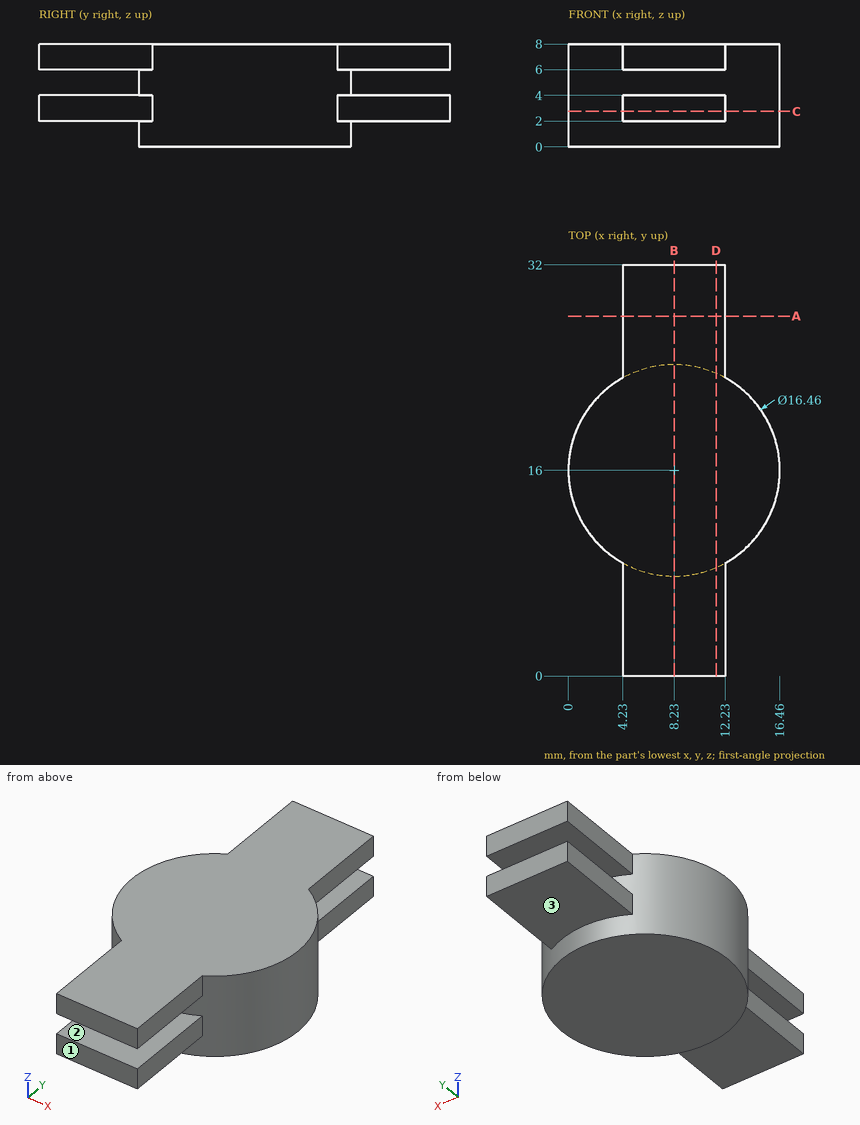
Geometry: see drawing. Coordinates: mm, zero at the bounding-box minimum. Give positions to 0.01 mm unless a question says otherwise; leave off trailing zeros. Write each loop counter-clockwise with the first axis right and the second up, starting at its lowest first coordinate (ties: lowest second). Pieces come first, ordered by that corner, then holes. Notation, with made-up numbers: M 51,74 L 65,74 A35 ccw 65,111 Z; hole C 87.25,0.25 d6. An arc over 180 degrees is marked long. Answer in a Markdown table with one row per item. Add a question column.
(1) Mould query, pull axis Z, two halves, no side actions, for the marked faces 1, 2 and 3. Classes: +Z half, -Z half, draft (parallel to the pull), parting line (faces both ways), or undercut.
(2) Section A-A on y = 28. Return loops of the section in (x, z).
(3) Section B-B on x = 8.23. Return loops of the section in (y, z), and give its area (3 significant figures).
(4) Section C-C on z = 2.75. Return loops of the section in (x, y).
(5) Section D-D on x = 11.5. Return loops of the section in (y, z).
(6) Ray query, line 1 (Z direction, x = 8, y = 25.5); line 2 (X direction, y = 29, z = 3); line 3 (Y direction, x = 8.25, z = 1.25). Return the intervals inside material, ascending.
(7) First-contact query: pin 1 (1.6 mm diameter, centred on y = 3.5, z = 7.5, fed in from +X); pin 2 (1 mm diameter, centred on y = 13.5, z = 1, fed in from +X); pin 3 (1.6 mm diameter, centred on y = 25.5, z = 3, fed in from -X); pin 4 (2 mm diameter, centred on x = 13.5, y = 25.5, fed in from +Z). Flat tips, straight axial feed; report the tip coordinate or a pass-through.
Result set:
| question | item | result |
|---|---|---|
| 1 | face 1 | draft |
| 1 | face 2 | undercut |
| 1 | face 3 | -Z half |
| 2 | outline | M 4.23,2 L 12.23,2 L 12.23,4 L 4.23,4 Z; M 4.23,6 L 12.23,6 L 12.23,8 L 4.23,8 Z |
| 3 | outline | M 0,2 L 7.77,2 L 7.77,0 L 24.23,0 L 24.23,2 L 32,2 L 32,4 L 24.23,4 L 24.23,6 L 32,6 L 32,8 L 0,8 L 0,6 L 7.77,6 L 7.77,4 L 0,4 Z |
| 3 | area | 194 mm^2 |
| 4 | outline | M 4.23,0 L 12.23,0 L 12.23,8.81 A8.23 ccw 12.23,23.19 L 12.23,32 L 4.23,32 L 4.23,23.19 A8.23 ccw 4.23,8.81 Z |
| 5 | outline | M 0,2 L 8.45,2 L 8.45,0 L 23.55,0 L 23.55,2 L 32,2 L 32,4 L 23.55,4 L 23.55,6 L 32,6 L 32,8 L 0,8 L 0,6 L 8.45,6 L 8.45,4 L 0,4 Z |
| 6 | line 1 | z = 2 to 4, 6 to 8 |
| 6 | line 2 | x = 4.23 to 12.23 |
| 6 | line 3 | y = 7.77 to 24.23 |
| 7 | pin 1 | stops at x = 12.23 |
| 7 | pin 2 | stops at x = 16.21 |
| 7 | pin 3 | stops at x = 4.23 |
| 7 | pin 4 | passes through |
